from build123d import *

# Parameters (mm, degrees)
EXTRUDE_START   = 0.2
SKETCH_1_R      = 6
SKETCH_1_R_2    = 3
EXTRUDE_1_DEPTH = 18.6
SKETCH_2_R      = 6.108417227
SKETCH_2_R_2    = 5.608417227
SKETCH_2_R_3    = 3.2
SKETCH_2_R_4    = 3
EXTRUDE_2_DEPTH = 19
FILLET_1_R      = 0.2


with BuildPart() as part:
    # 草图1 → 凸台-拉伸1 (new body)
    with BuildSketch(Plane(origin=(0, 0, 0), x_dir=(1, 0, 0), z_dir=(0, 1, 0)).offset(EXTRUDE_START)):
        with Locations(Location((0, 0, 0), (0, 0, 270))):
            Circle(SKETCH_1_R)
        with Locations(Location((0, 0, 0), (0, 0, 270))):
            Circle(SKETCH_1_R_2, mode=Mode.SUBTRACT)
    extrude(amount=EXTRUDE_1_DEPTH)

    # 草图2 → 凸台-拉伸2 (add)
    # profile 1 of 2: a face of its own
    with BuildSketch(Plane(origin=(0, 0, 0), x_dir=(1, 0, 0), z_dir=(0, 1, 0))):
        with Locations(Location((0, 0, 0), (0, 0, 270))):
            Circle(SKETCH_2_R)
        with Locations(Location((0, 0, 0), (0, 0, 270))):
            Circle(SKETCH_2_R_2, mode=Mode.SUBTRACT)
    # profile 2 of 2: a face of its own
    with BuildSketch(Plane(origin=(0, 0, 0), x_dir=(1, 0, 0), z_dir=(0, 1, 0))):
        with Locations(Location((0, 0, 0), (0, 0, 270))):
            Circle(SKETCH_2_R_3)
        with Locations(Location((0, 0, 0), (0, 0, 270))):
            Circle(SKETCH_2_R_4, mode=Mode.SUBTRACT)
    extrude(amount=EXTRUDE_2_DEPTH)

    # 圆角1
    fillet_1_edges = [part.edges().sort_by_distance(p)[0] for p in [
        (0, 0, -6.108417227),
        (0, 19, -6.108417227),
        (0, 0, -3.2),
        (0, 19, -3.2),
    ]]
    fillet(fillet_1_edges, radius=FILLET_1_R - 0.0001)  # a hair under: the kernel refuses the full size


solid = part.part
The model under review builds one solid part; all positions refer to its coordinate system, in mm. Coordinates: 2 decimals unless noted, no trailing zeros. Loops run counter-clockwise (first coordinate to the right, second up) from the corner with the lowest first, then second, coordinate; pieces in that order, holes last. Notation, with made-up numbers: (-23.5, 67.25) -> (16.5, 67.25) arc R4 cw to (16.5, 72.25) -> close; hole circle Ø4 at (20, 87). An arc over 180 degrees is marked (long way). Use a Markdown table: item, result. Add a question column.
1. Draft analysis for pull direction Z (two halves, no side actions). For faces 1 (the face through (-2.4, 0.2, 2.4)), 2 (the face through (0.9, 9.37, 2.86)), 3 (the face through (-3.717, 9.37, -4.847)), state which applies: pulls with the +Z half, pulls with the -Z half, needs draft (parallel to the pull), parting line crosses it, or undercut.
2. Add section C-C on y = 7.25. Write out the cut boundary in (x, z).
3. Clearance check with flat-ended pins moving along their axes: pin 1 Ø3 at (x, y) = (2, 13.5) entering from +Z; pin 2 Ø4 at (x, z) = (3.5, 0) entering from +Y; pin 3 Ø3 at (x, y) = (-3, 5) entering from +Z; pin 4 Ø2 at (x, z) = (2.5, -3.5) entering from -Y. State where each tip first meets the part, or that it passes through.
4. To check wall thickness, follow line 1 (X direction, y = 14, z = 0); line 2 (Y direction, x = 3.25, z = -4); line 3 (Z direction, x = -1.75, y = 16.5). State the ranges of each line that lie inside material, in increasing order.
Returned:
| question | item | result |
|---|---|---|
| 1 | face 1 | undercut |
| 1 | face 2 | undercut |
| 1 | face 3 | parting line crosses it |
| 2 | outline | circle Ø12.22 at (0, 0); hole circle Ø6 at (0, 0) |
| 3 | pin 1 | stops at z = 6.09 |
| 3 | pin 2 | stops at y = 19 |
| 3 | pin 3 | stops at z = 5.92 |
| 3 | pin 4 | stops at y = 0.2 |
| 4 | line 1 | x = -6.11 to -3, 3 to 6.11 |
| 4 | line 2 | y = 0.2 to 18.8 |
| 4 | line 3 | z = -5.85 to -2.44, 2.44 to 5.85 |
